from build123d import *

# Parameters (mm, degrees)
BOSS_EXTRU_1_DEPTH      = 35
ESQUISSE3_W             = 15.551416147
ESQUISSE3_H             = 5
BOSS_EXTRU_3_DEPTH      = 3.5
ESQUISSE4_W             = 14.990100516
ESQUISSE4_H             = 8.543070591
ENL_V_MAT_EXTRU_4_DEPTH = 11
ESQUISSE5_W             = 2.711143337
ESQUISSE5_H             = 4.509933932
BOSS_EXTRU_4_DEPTH      = 3.5
CONG_2_R                = 0.1
ENL_V_MAT_EXTRU_7_DEPTH = 11


with BuildPart() as part:
    # Esquisse1 → Boss.-Extru.1 (new body)
    with BuildSketch(Plane.XY):
        Polygon((0, -0.638190255), (-5.531744574, 4.893554319), (10.018583778, 4.709618574), (10.016881657, -6.092719993), (-3.032142088, -0.792171418), (0, -1.326819878), align=None)
    extrude(amount=BOSS_EXTRU_1_DEPTH)

    # Esquisse3 → Boss.-Extru.3 (add)
    with BuildSketch(Plane(origin=(0.05710105, 4.827447131, 0), x_dir=(0.9999300516333419, -0.011827588111794733, 0), z_dir=(0.011827588111794733, 0.9999300516333419, 0))):
        with Locations((2.186471492, -32.5)):
            Rectangle(ESQUISSE3_W, ESQUISSE3_H)
    extrude(amount=BOSS_EXTRU_3_DEPTH)

    # Esquisse4 → Enlèv. mat.-Extru.4 (cut)
    with BuildSketch(Plane(origin=(0.21677349, 18.326502828, 0), x_dir=(0.9999300516333419, -0.011827588111794735, 0), z_dir=(0.011827588111794735, 0.9999300516333419, 0))):
        with Locations((5.405813676, -32.865617066)):
            Rectangle(ESQUISSE4_W, ESQUISSE4_H)
    extrude(amount=-ENL_V_MAT_EXTRU_4_DEPTH, mode=Mode.SUBTRACT)

    # Esquisse5 → Boss.-Extru.4 (add)
    with BuildSketch(Plane(origin=(0.05710105, 4.827447131, 0), x_dir=(0.9999300516333419, -0.011827588111794733, 0), z_dir=(0.011827588111794733, 0.9999300516333419, 0))):
        with Locations((-4.233664914, -2.254966966)):
            Rectangle(ESQUISSE5_W, ESQUISSE5_H)
    extrude(amount=BOSS_EXTRU_4_DEPTH)

    # Congé2
    cong_2_edges = [part.edges().sort_by_distance(p)[0] for p in [
        (-3.032142088, -0.792171418, 17.5),
    ]]
    fillet(cong_2_edges, radius=CONG_2_R)

    # Esquisse6 → Enlèv. mat.-Extru.7 (cut)
    with BuildSketch(Plane(origin=(-4.469048391, -11.002015687, 0), x_dir=(-0.9264818598701292, 0.37633942569386236, 0), z_dir=(-0.37633942569386236, -0.9264818598701292, 0))):
        Polygon((1.67530136, 0.492691421), (1.67530136, -38.461342547), (0.532077108, 0.492691421), align=None)
    extrude(amount=-ENL_V_MAT_EXTRU_7_DEPTH, mode=Mode.SUBTRACT)


solid = part.part
Input: part model. Units: mm. Frame: model coordinates. A direction names the side the tool comes from. Coordinates: 2 decimals unless noted, no trailing zeros. Loops run counter-clockwise (first coordinate to the right, second up) from the corner with the lowest first, then second, coordinate; pieces in that order, holes last. Notation, with made-up numbers: (86.25, -20) -> (112.25, -20) arc R18 ccw to (112.25, 3) -> close; hole circle Ø3 at (42, 36). An arc over 180 degrees is marked (long way). Write item = value, one per line. Start each with the question number.
Item 1: Cut plane B-B, the plane x = -0.5. Return loops of the section in (y, z).
Item 2: Reachability of faces 1 (the face through (4, 1, 0)), 2 (the face through (-4, 7, 4.51)) from +Z, -Z, +X, -X, +Y, -Y: full face, straight path, thin tool, end or side. Return the list, or none.
Item 3: Material intervals for line 1 (Z direction, x = 8.75, y = 6); line 2 (Y direction, x = -0.25, z = 23); line 3 (X direction, y = 5.25, z = 3), sorted ascending.
Item 4: Cut plane C-C, the plane z = 13. Return loops of the section in (x, y), plus the area to 3 significant figures.
Item 5: Mould query, pull axis Y, two halves, no side actions, for faces 3 (the face through (4, 3, 35)), 4 (the face through (-0.83, -1.18, 17.26)), 5 (the face through (-2.73, 2.09, 17.26)), 6 (the face through (4.014, -3.655, 17.255)). Classes: pulls with the +Y half, pulls with the -Y half, needs draft (parallel to the pull), parting line crosses it, or undercut.
Item 6: Cut plane D-D, the plane x = 2.5. Return loops of the section in (y, z), plus the area to 3 significant figures.
Item 7: First-contact query: P1, Ø8, axis at x = 3.5, z = 13, coming from the -Y side; P2, Ø3, axis at y = 0, z = 12, coming from the +X side; P3, Ø1.1, axis at x = 0.5, y = 7, coming from the -Z side. Flat tips, straight axial feed; report the tip coordinate or a pass-through.
Item 8: Cut plane A-A, the plane y = 6.75. Return loops of the section in (x, z).
Ans:
q1.outline = (-1.82, 0) -> (-1.24, 0) -> (-1.24, 35) -> (-1.82, 35) -> close; (-0.14, 0) -> (4.83, 0) -> (4.83, 30) -> (7.33, 30) -> (7.33, 35) -> (-0.14, 35) -> close
q2.face_1 = -Z, +X, -X, +Y, -Y
q2.face_2 = +X, -X, +Y
q3.line_1 = 30 to 35
q3.line_2 = -1.92 to -1.28, -0.39 to 4.83
q3.line_3 = -5.53 to -2.82
q4.outline = (-5.53, 4.89) -> (0, -0.64) -> (0, -1.33) -> (-1.44, -1.07) -> (-1.57, -1.39) -> (10.02, -6.09) -> (10.02, 4.71) -> close
q4.area = 104 mm²
q5.face_3 = needs draft
q5.face_4 = undercut
q5.face_5 = undercut
q5.face_6 = pulls with the -Y half
q6.outline = (-3.04, 0) -> (4.8, 0) -> (4.8, 30) -> (7.3, 30) -> (7.3, 35) -> (-3.04, 35) -> close
q6.area = 287 mm²
q7.P1 = -5.07
q7.P2 = 10.02
q7.P3 = 30
q8.outline = (-5.51, 0) -> (-2.8, 0) -> (-2.8, 4.51) -> (-5.51, 4.51) -> close; (-5.51, 30) -> (10.04, 30) -> (10.04, 35) -> (-5.51, 35) -> close
